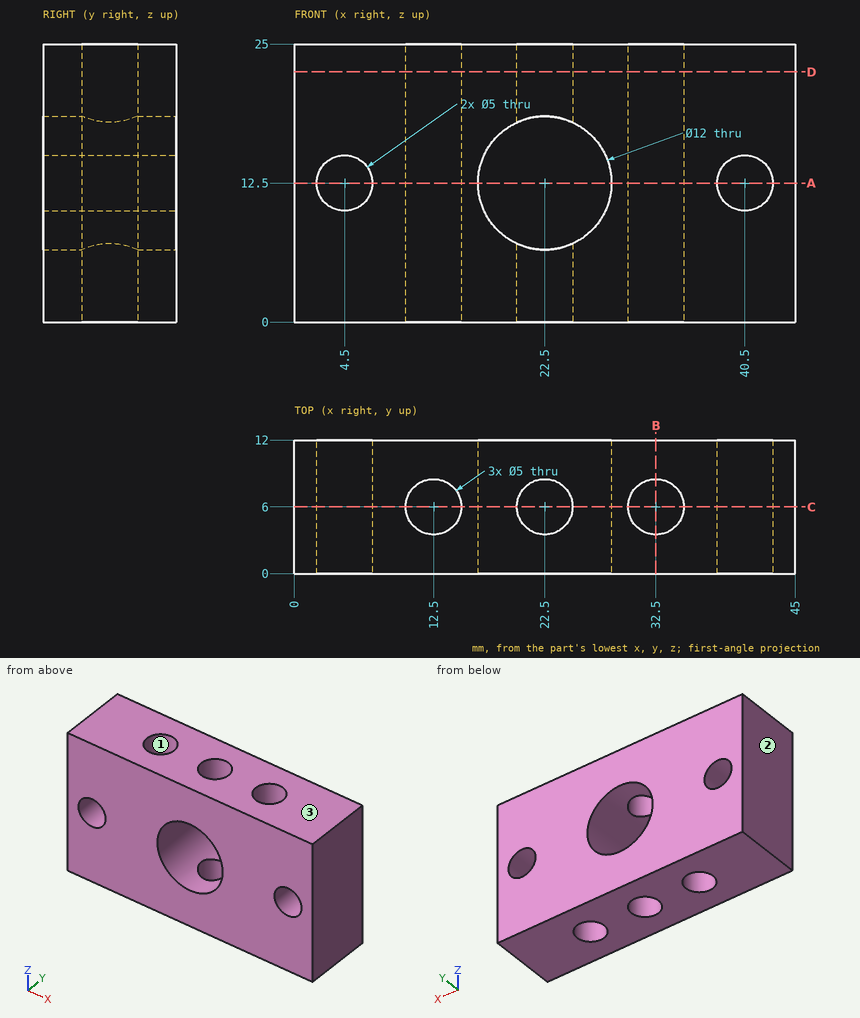
Input: dimensioned drawing with shaded views. Units: mm. Origin: part minimum x, y, z. Coordinates: 2 decimals unless noted, no trailing zeros. Order: outer loops, then holes, each group sorted by start corner. A loop starts at its lowest first (then second) coordinate and runs counter-clockwise, first axis right, second up. Notation, with made-up numbers: M -24.5,11 L 10.5,11 A9 cw 10.5,24 Z; hole C -9,-36.5 d5. An arc over 180 degrees is marked long. Write each question's results on one line, items separated by ' | '. Start each with the question number.
Item 1: Draft query along X for the marked faces 1, 2 and 3. Return one class per face: pulls with the +X half, pulls with the -X half, needs draft (parallel to the pull), parting line crosses it, or undercut.
Item 2: Line query: probe 1 along Z at (x, y) = (40.5, 6.25); probe 2 along Y at (x, z) = (12.5, 11); probe 3 along Z at (x, y) = (25, 2). Output: solid intervals per line, ascending.
Item 3: Cut plane C-C (y = 6). Return loops of the section in (x, z).
Item 4: Cut plane B-B (x = 32.5). Return loops of the section in (y, z), and give its area (3 significant figures).
Item 5: Cut plane A-A (z = 12.5). Return loops of the section in (x, y), and give its area (3 significant figures).
Item 6: Cut plane D-D (z = 22.5). Return loops of the section in (x, y).
Checked values:
1) face 1: undercut | face 2: pulls with the -X half | face 3: needs draft
2) probe 1: z = 0 to 10, 15 to 25 | probe 2: y = 0 to 3.5, 8.5 to 12 | probe 3: z = 0 to 7.05, 17.95 to 25
3) outline: M 0,0 L 10,0 L 10,25 L 0,25 Z; M 15,0 L 20,0 L 20,7.05 A6 cw 20,17.95 L 20,25 L 15,25 Z; M 25,0 L 30,0 L 30,25 L 25,25 L 25,17.95 A6 cw 25,7.05 Z; M 35,0 L 45,0 L 45,25 L 35,25 Z; hole C 4.5,12.5 d5; hole C 40.5,12.5 d5
4) outline: M 0,0 L 3.5,0 L 3.5,25 L 0,25 Z; M 8.5,0 L 12,0 L 12,25 L 8.5,25 Z | area: 175 mm2
5) outline: M 0,0 L 2,0 L 2,12 L 0,12 Z; M 7,0 L 16.5,0 L 16.5,12 L 7,12 Z; M 28.5,0 L 38,0 L 38,12 L 28.5,12 Z; M 43,0 L 45,0 L 45,12 L 43,12 Z; hole C 12.5,6 d5; hole C 32.5,6 d5 | area: 237 mm2
6) outline: M 0,0 L 45,0 L 45,12 L 0,12 Z; hole C 12.5,6 d5; hole C 22.5,6 d5; hole C 32.5,6 d5
